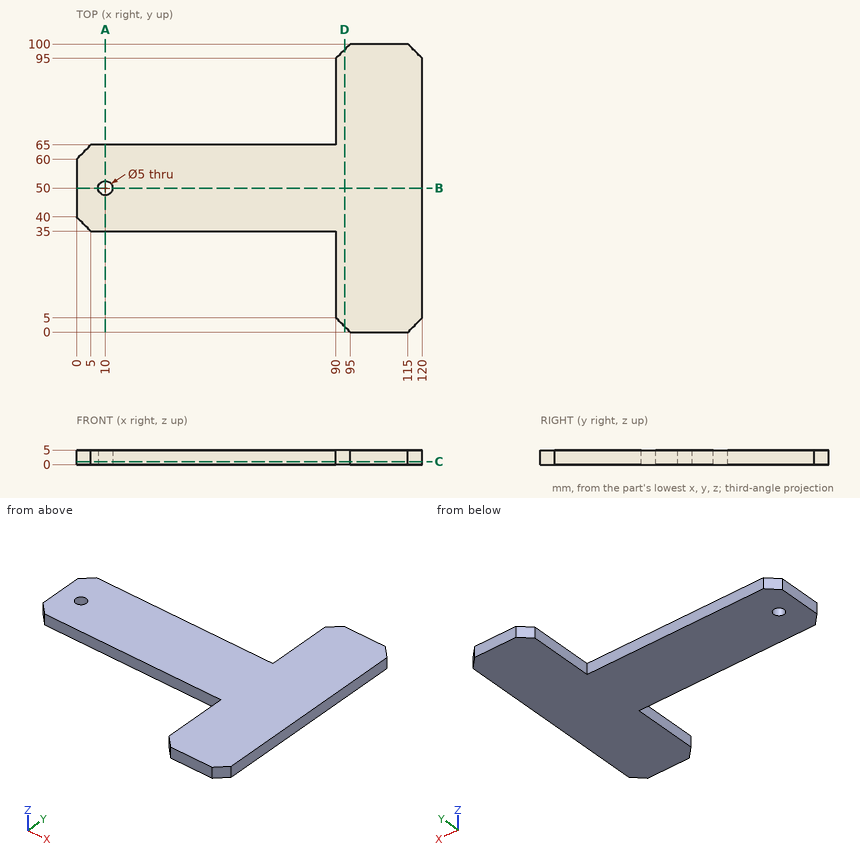
Geometry: see drawing. Coordinates: mm, zero at the bounding-box minimum. Give positions to 0.01 mm unless a question says otherwise; leave off trailing zeros. Write each loop counter-clockwise with the first axis right and the second up, starting at its lowest first coordinate (ties: lowest second). Pieces come first, ordered by that corner, then holes. Notation, with made-up numbers: M 67.5,72.5 L 100.5,72.5 A15 cw 100.5,82.5 Z; hole C -36.75,-11.5 d4. An arc over 180 degrees is marked long. Return JSON: item names as keys, results as strings. Group by question number.
1) Cut plane D-D, the plane x = 93. Output: boundary loops of the cut face in (y, z).
2) Cut plane A-A, the plane x = 10. Output: boundary loops of the cut face in (y, z), then the cut area to 3 significant figures.
3) Cut plane B-B, the plane y = 50. Output: boundary loops of the cut face in (x, z).
4) Cut plane C-C, the plane z = 1. Output: boundary loops of the cut face in (x, y).
5) First-contact query: pin 1 Ø1.5 at (x, z) = (63.5, 3) entering from +Y; pin 2 Ø3 at (y, z) = (87.5, 1.5) entering from -X. Flat tips, straight axial feed; report the tip coordinate or a pass-through.
6) Ray query, L1, parallel to X at y = 50, z = 3.45; L2, parallel to Y at x = 10, z = 4; L3, parallel to Y at x = 86.5, z = 3.2. Return the intervals inside material, ascending.
Data:
{
 "1": {"outline": "M 2,0 L 98,0 L 98,5 L 2,5 Z"},
 "2": {"outline": "M 35,0 L 47.5,0 L 47.5,5 L 35,5 Z; M 52.5,0 L 65,0 L 65,5 L 52.5,5 Z", "area": "125 mm²"},
 "3": {"outline": "M 0,0 L 7.5,0 L 7.5,5 L 0,5 Z; M 12.5,0 L 120,0 L 120,5 L 12.5,5 Z"},
 "4": {"outline": "M 0,40 L 5,35 L 90,35 L 90,5 L 95,0 L 115,0 L 120,5 L 120,95 L 115,100 L 95,100 L 90,95 L 90,65 L 5,65 L 0,60 Z; hole C 10,50 d5"},
 "5": {"pin 1": "stops at y = 65", "pin 2": "stops at x = 90"},
 "6": {"L1": "x = 0 to 7.5, 12.5 to 120", "L2": "y = 35 to 47.5, 52.5 to 65", "L3": "y = 35 to 65"}
}
